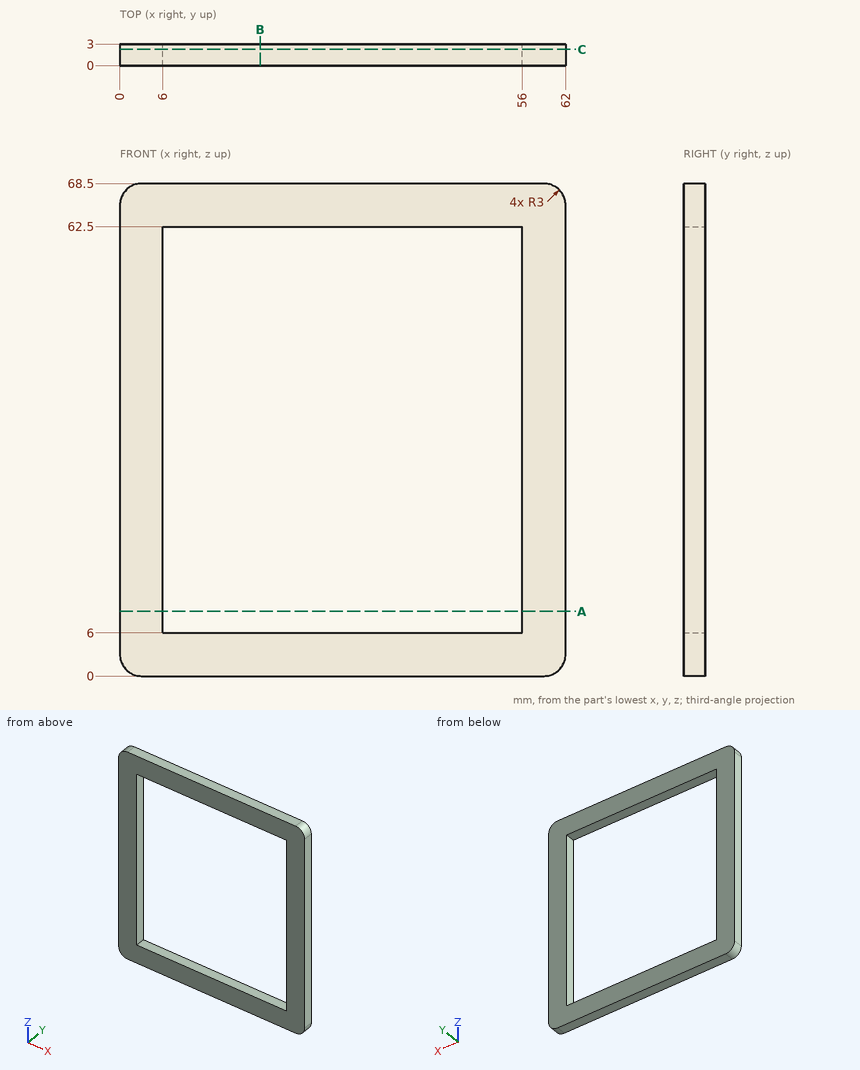
Here's the drawing with two shaded views (mm, measured from the low corner). I have some questions. Round coordinates to 2 decimals unless told otherwise and drop trailing zeros. Order: outer loops, then holes, each group sorted by start corner. A loop starts at its lowest first (then second) coordinate and runs counter-clockwise, first axis right, second up. Notation, with made-up numbers: (6, 71) -> (23, 71) arc R28 ccw to (23, 97) -> close; hole circle Ø4 at (-21, -17.5). An arc over 180 degrees is marked (long way). Write each question's results on one line, items separated by ' | '. Start each with the question number.
Item 1: If we section it at C-C, the plane y = 2.25: Write out the boundary of the cut face in (x, z), then the cut area to 3 significant figures.
Item 2: If we section it at B-B, the plane x = 19.5: Write out the boundary of the cut face in (y, z).
Item 3: Please list where these lines run through material, in increasing order: L1, parallel to X at y = 0.55, z = 43; L2, parallel to Z at x = 10, y = 1.35.
Item 4: If we section it at A-A, the plane z = 9: Write out the boundary of the cut face in (x, y).
Results:
1) outline: (0, 3) arc R3 ccw to (3, 0) -> (59, 0) arc R3 ccw to (62, 3) -> (62, 65.5) arc R3 ccw to (59, 68.5) -> (3, 68.5) arc R3 ccw to (0, 65.5) -> close; hole (6, 6) -> (56, 6) -> (56, 62.5) -> (6, 62.5) -> close | area: 1,410 mm2
2) outline: (0, 0) -> (3, 0) -> (3, 6) -> (0, 6) -> close; (0, 62.5) -> (3, 62.5) -> (3, 68.5) -> (0, 68.5) -> close
3) L1: x = 0 to 6, 56 to 62 | L2: z = 0 to 6, 62.5 to 68.5
4) outline: (0, 0) -> (6, 0) -> (6, 3) -> (0, 3) -> close; (56, 0) -> (62, 0) -> (62, 3) -> (56, 3) -> close
